```python
from build123d import *

# Parameters (mm, degrees)
BOSS_EXTRU_1_DEPTH      = 12
BOSS_EXTRU_1_DEPTH_BACK = 12
ENL_V_START             = 9
ESQUISSE2_R             = 1
ENL_V_MAT_EXTRU_1_DEPTH = 4
CONG_1_R                = 1


with BuildPart() as part:
    # Esquisse1 → Boss.-Extru.1 (new body, two sides)
    with BuildSketch(Plane.XY) as boss_extru_1_sk:
        with BuildLine():
            Line((11, -9), (2.692582404, -9))
            ThreePointArc((2.692582404, -9), (0, 5.5), (-2.692582404, -9))
            Line((-2.692582404, -9), (-11, -9))
            Line((-11, -9), (-11, 9))
            Line((-11, 9), (11, 9))
            Line((11, 9), (11, -9))
        make_face()
    extrude(amount=BOSS_EXTRU_1_DEPTH)
    extrude(boss_extru_1_sk.sketch, amount=-BOSS_EXTRU_1_DEPTH_BACK)

    # Esquisse2 → Enlèv. mat.-Extru.1 (cut)
    with BuildSketch(Plane(origin=(0, 0, 0), x_dir=(1, 0, 0), z_dir=(0, 1, 0)).offset(ENL_V_START)):
        with Locations((-7, 8)):
            Circle(ESQUISSE2_R)
        with Locations((7, 8)):
            Circle(ESQUISSE2_R)
        with Locations((7, -8)):
            Circle(ESQUISSE2_R)
        with Locations((-7, -8)):
            Circle(ESQUISSE2_R)
    extrude(amount=-ENL_V_MAT_EXTRU_1_DEPTH, mode=Mode.SUBTRACT)

    # Congé1
    cong_1_edges = [part.edges().sort_by_distance(p)[0] for p in [
        (-11, 9, 0),
        (11, 9, 0),
        (11, -9, 0),
        (2.692582404, -9, 0),
        (-2.692582404, -9, 0),
        (-11, -9, 0),
        (0, 5.5, -12),
        (6.846291202, -9, -12),
        (-11, 0, 12),
        (-6.846291202, -9, 12),
        (0, 5.5, 12),
        (6.846291202, -9, 12),
        (11, 0, 12),
        (0, 9, 12),
        (11, 0, -12),
        (0, 9, -12),
        (-11, 0, -12),
        (-6.846291202, -9, -12),
    ]]
    fillet(cong_1_edges, radius=CONG_1_R)


solid = part.part
```
The model under review builds one solid part; all positions refer to its coordinate system, in mm. A direction names the side the tool comes from. Round coordinates to 2 decimals unless told otherwise and drop trailing zeros. Write each loop counter-clockwise with the first axis right and the second up, starting at its lowest first coordinate (ties: lowest second). Pieces come first, ordered by that corner, then holes. Notation, with made-up numbers: (21.25, 25) -> (47.25, 25) arc R11 cw to (47.25, 35) -> close; hole circle Ø9 at (-14.75, 22.25). An arc over 180 degrees is marked (long way). Use CSV: the item, a comma, the result in double quotes.
Q1. To check wall thickness, follow probe 1 along X at (y, z) = (7.95, 8); probe 2 along Z at (x, y) = (7, 6.45); probe 3 along X at (y, z) = (-8, -1). State the ranges of each line that lie inside material, in increasing order. Write a range as [from, to].
Checks:
probe 1,"[-11, -8], [-6, 6], [8, 11]"
probe 2,"[-12, -9], [-7, 7], [9, 12]"
probe 3,"[-11, -5.02], [5.02, 11]"
Q2. For pin 1 Ø2 at (x, z) = (6.5, 8) entering from +Y; pin 2 Ø6 at (x, y) = (1.5, -2) entering from +Z (3 decimals), all flat-tipped, find the tip position at first contact; note any pin that passes through.
Checks:
pin 1,"y = 9"
pin 2,"through"
Q3. Consider section B-B (z = -8.5). Give the boundary of the cut face in (x, y), then the cut area to 3 significant figures.
Checks:
outline,"(-11, -8) arc R1 ccw to (-10, -9) -> (-6.02, -9) arc R1 ccw to (-5.31, -7.29) arc R7.5 cw (long way) to (5.31, -7.29) arc R1 ccw to (6.02, -9) -> (10, -9) arc R1 ccw to (11, -8) -> (11, 8) arc R1 ccw to (10, 9) -> (7.87, 9) -> (7.87, 5) -> (6.13, 5) -> (6.13, 9) -> (-6.13, 9) -> (-6.13, 5) -> (-7.87, 5) -> (-7.87, 9) -> (-10, 9) arc R1 ccw to (-11, 8) -> close"
area,"203 mm²"
Q4. Consider section A-A (x = 0). Give the boundary of the cut face in (y, z).
Checks:
outline,"(5.5, -11) arc R1 ccw to (6.5, -12) -> (8, -12) arc R1 ccw to (9, -11) -> (9, 11) arc R1 ccw to (8, 12) -> (6.5, 12) arc R1 ccw to (5.5, 11) -> close"
Q5. Consider section C-C (z = 8). Give the boundary of the cut face in (x, y), then the cut area to 3 significant figures.
Checks:
outline,"(-11, -8) arc R1 ccw to (-10, -9) -> (-6.02, -9) arc R1 ccw to (-5.31, -7.29) arc R7.5 cw (long way) to (5.31, -7.29) arc R1 ccw to (6.02, -9) -> (10, -9) arc R1 ccw to (11, -8) -> (11, 8) arc R1 ccw to (10, 9) -> (8, 9) -> (8, 5) -> (6, 5) -> (6, 9) -> (-6, 9) -> (-6, 5) -> (-8, 5) -> (-8, 9) -> (-10, 9) arc R1 ccw to (-11, 8) -> close"
area,"201 mm²"
Q6. For faces 1 (the cylindrical face through (-7, 7, 7)), 2 (the cylindrical face through (-10.699, 0.112, -11.715)), list the 3-axis set-ups (+Z, -Z, +X, -X, +Y, -Y) from which the entire face can be reached by the end or side of a thin tool; tool diameter is ignored.
Checks:
face 1,"+Y"
face 2,"-Z, -X, +Y, -Y"
Q7. Mouldability with a two-part tool opening along Y and no side actions: class faces 3 (the cylindrical face through (5.104, -8.399, -0.154)), 4 (the flat face through (0, 9, 0)), 5 (the cylindrical face through (7.983, -8.715, 11.699)), 6 (the cylindrical face through (-5.09, -8.37, -0.15)) as released by +Y, released by -Y, zero draft, split by the parting line, or undercut.
Checks:
face 3,"undercut"
face 4,"released by +Y"
face 5,"released by -Y"
face 6,"undercut"
